Verification items for the finished model (mm, model axes). Round coordinates to 2 decimals unless told otherwise and drop trailing zeros. Loops run counter-clockwise (first coordinate to the right, second up) from the corner with the lowest first, then second, coordinate; pieces in that order, holes last. Notation, with made-up numbers: (-2, 68.5) - (33, 68.5) arc R27 ccw to (33, 90.5) - close; hole circle Ø3 at (79.5, -15.75). An arc over 180 degrees is marked (long way). Use a Markdown table: item, result. Add a question column.
```python
from build123d import *

# Parameters (mm, degrees)
SKETCH1_W          = 187.325
SKETCH1_H          = 332.057083461
EXTRUDE1_DEPTH     = 4.7625
CUT_EXTRUDE1_REACH = 264.098
CUT_EXTRUDE2_REACH = 264.098
SKETCH3_R          = 47.625
SKETCH3_R_2        = 8.5328125
FILLET1_R          = 6.35
CUT_EXTRUDE3_REACH = 264.098
SKETCH4_W          = 4.7625
SKETCH4_H          = 98.425


with BuildPart() as part:
    # Sketch1 → Extrude1 (new body)
    with BuildSketch(Plane.XY):
        with Locations((0, -78.716041731)):
            Rectangle(SKETCH1_W, SKETCH1_H)
    extrude(amount=-EXTRUDE1_DEPTH)

    # Sketch2 → Cut-Extrude1 (cut, up to next)
    with BuildSketch(Plane.XY, mode=Mode.PRIVATE) as cut_extrude1_sk1:
        with BuildLine():
            Line((-22.225, -203.2), (-22.225, -177.8))
            ThreePointArc((-22.225, -177.8), (0, -155.575), (22.225, -177.8))
            Line((22.225, -177.8), (22.225, -203.2))
            ThreePointArc((22.225, -203.2), (0, -225.425), (-22.225, -203.2))
        make_face()
    cut_extrude1_tool1 = extrude(cut_extrude1_sk1.sketch, amount=-CUT_EXTRUDE1_REACH, mode=Mode.PRIVATE) & part.part
    # Sketch2 → Cut-Extrude1 (cut, up to next)
    with BuildSketch(Plane.XY, mode=Mode.PRIVATE) as cut_extrude1_sk2:
        with BuildLine():
            Line((49.99355, -108.9152), (49.99355, -134.3152))
            ThreePointArc((49.99355, -134.3152), (46.0248, -138.28395), (42.05605, -134.3152))
            Line((42.05605, -134.3152), (42.05605, -108.9152))
            ThreePointArc((42.05605, -108.9152), (46.0248, -104.94645), (49.99355, -108.9152))
        make_face()
    cut_extrude1_tool2 = extrude(cut_extrude1_sk2.sketch, amount=-CUT_EXTRUDE1_REACH, mode=Mode.PRIVATE) & part.part
    # Sketch2 → Cut-Extrude1 (cut, up to next)
    with BuildSketch(Plane.XY, mode=Mode.PRIVATE) as cut_extrude1_sk3:
        with BuildLine():
            Line((-42.05605, -108.9152), (-42.05605, -134.3152))
            ThreePointArc((-42.05605, -134.3152), (-46.0248, -138.28395), (-49.99355, -134.3152))
            Line((-49.99355, -134.3152), (-49.99355, -108.9152))
            ThreePointArc((-49.99355, -108.9152), (-46.0248, -104.94645), (-42.05605, -108.9152))
        make_face()
    cut_extrude1_tool3 = extrude(cut_extrude1_sk3.sketch, amount=-CUT_EXTRUDE1_REACH, mode=Mode.PRIVATE) & part.part
    # Sketch2 → Cut-Extrude1 (cut, up to next)
    with BuildSketch(Plane.XY, mode=Mode.PRIVATE) as cut_extrude1_sk4:
        with BuildLine():
            Line((49.99355, -200.9648), (49.99355, -226.3648))
            ThreePointArc((49.99355, -226.3648), (46.0248, -230.33355), (42.05605, -226.3648))
            Line((42.05605, -226.3648), (42.05605, -200.9648))
            ThreePointArc((42.05605, -200.9648), (46.0248, -196.99605), (49.99355, -200.9648))
        make_face()
    cut_extrude1_tool4 = extrude(cut_extrude1_sk4.sketch, amount=-CUT_EXTRUDE1_REACH, mode=Mode.PRIVATE) & part.part
    # Sketch2 → Cut-Extrude1 (cut, up to next)
    with BuildSketch(Plane.XY, mode=Mode.PRIVATE) as cut_extrude1_sk5:
        with BuildLine():
            Line((-42.05605, -200.9648), (-42.05605, -226.3648))
            ThreePointArc((-42.05605, -226.3648), (-46.0248, -230.33355), (-49.99355, -226.3648))
            Line((-49.99355, -226.3648), (-49.99355, -200.9648))
            ThreePointArc((-49.99355, -200.9648), (-46.0248, -196.99605), (-42.05605, -200.9648))
        make_face()
    cut_extrude1_tool5 = extrude(cut_extrude1_sk5.sketch, amount=-CUT_EXTRUDE1_REACH, mode=Mode.PRIVATE) & part.part
    add(cut_extrude1_tool1.solids().sort_by_distance((0, -190.5, 0))[0], mode=Mode.SUBTRACT)
    add(cut_extrude1_tool2.solids().sort_by_distance((46.0248, -121.6152, 0))[0], mode=Mode.SUBTRACT)
    add(cut_extrude1_tool3.solids().sort_by_distance((-46.0248, -121.6152, 0))[0], mode=Mode.SUBTRACT)
    add(cut_extrude1_tool4.solids().sort_by_distance((46.0248, -213.6648, 0))[0], mode=Mode.SUBTRACT)
    add(cut_extrude1_tool5.solids().sort_by_distance((-46.0248, -213.6648, 0))[0], mode=Mode.SUBTRACT)

    # Sketch3 → Cut-Extrude2 (cut, up to next)
    with BuildSketch(Plane(origin=(0, 0, 0), x_dir=(-1, 0, 0), z_dir=(0, 0, -1)), mode=Mode.PRIVATE) as cut_extrude2_sk1:
        Circle(SKETCH3_R)
    cut_extrude2_tool1 = extrude(cut_extrude2_sk1.sketch, amount=CUT_EXTRUDE2_REACH, mode=Mode.PRIVATE) & part.part
    # Sketch3 → Cut-Extrude2 (cut, up to next)
    with BuildSketch(Plane(origin=(0, 0, 0), x_dir=(-1, 0, 0), z_dir=(0, 0, -1)), mode=Mode.PRIVATE) as cut_extrude2_sk2:
        with Locations((65.0875, 65.0875)):
            Circle(SKETCH3_R_2)
    cut_extrude2_tool2 = extrude(cut_extrude2_sk2.sketch, amount=CUT_EXTRUDE2_REACH, mode=Mode.PRIVATE) & part.part
    # Sketch3 → Cut-Extrude2 (cut, up to next)
    with BuildSketch(Plane(origin=(0, 0, 0), x_dir=(-1, 0, 0), z_dir=(0, 0, -1)), mode=Mode.PRIVATE) as cut_extrude2_sk3:
        with Locations((-65.0875, 65.0875)):
            Circle(SKETCH3_R_2)
    cut_extrude2_tool3 = extrude(cut_extrude2_sk3.sketch, amount=CUT_EXTRUDE2_REACH, mode=Mode.PRIVATE) & part.part
    # Sketch3 → Cut-Extrude2 (cut, up to next)
    with BuildSketch(Plane(origin=(0, 0, 0), x_dir=(-1, 0, 0), z_dir=(0, 0, -1)), mode=Mode.PRIVATE) as cut_extrude2_sk4:
        with Locations((-65.0875, -65.0875)):
            Circle(SKETCH3_R_2)
    cut_extrude2_tool4 = extrude(cut_extrude2_sk4.sketch, amount=CUT_EXTRUDE2_REACH, mode=Mode.PRIVATE) & part.part
    # Sketch3 → Cut-Extrude2 (cut, up to next)
    with BuildSketch(Plane(origin=(0, 0, 0), x_dir=(-1, 0, 0), z_dir=(0, 0, -1)), mode=Mode.PRIVATE) as cut_extrude2_sk5:
        with Locations((65.0875, -65.0875)):
            Circle(SKETCH3_R_2)
    cut_extrude2_tool5 = extrude(cut_extrude2_sk5.sketch, amount=CUT_EXTRUDE2_REACH, mode=Mode.PRIVATE) & part.part
    add(cut_extrude2_tool1.solids().sort_by_distance((0, 0, 0))[0], mode=Mode.SUBTRACT)
    add(cut_extrude2_tool2.solids().sort_by_distance((-65.0875, 65.0875, 0))[0], mode=Mode.SUBTRACT)
    add(cut_extrude2_tool3.solids().sort_by_distance((65.0875, 65.0875, 0))[0], mode=Mode.SUBTRACT)
    add(cut_extrude2_tool4.solids().sort_by_distance((65.0875, -65.0875, 0))[0], mode=Mode.SUBTRACT)
    add(cut_extrude2_tool5.solids().sort_by_distance((-65.0875, -65.0875, 0))[0], mode=Mode.SUBTRACT)

    # Fillet1
    fillet1_edges = [part.edges().sort_by_distance(p)[0] for p in [
        (93.6625, -244.744583461, -2.38125),
        (-93.6625, -244.744583461, -2.38125),
        (-93.6625, 87.3125, -2.38125),
        (93.6625, 87.3125, -2.38125),
    ]]
    fillet(fillet1_edges, radius=FILLET1_R)

    # Sketch4 → Cut-Extrude3 (cut, up to next)
    with BuildSketch(Plane(origin=(0, 0, -4.7625), x_dir=(-1, 0, 0), z_dir=(0, 0, -1)), mode=Mode.PRIVATE) as cut_extrude3_sk1:
        with Locations((-91.28125, 0)):
            Rectangle(SKETCH4_W, SKETCH4_H)
    cut_extrude3_tool1 = extrude(cut_extrude3_sk1.sketch, amount=-CUT_EXTRUDE3_REACH, mode=Mode.PRIVATE) & part.part
    # Sketch4 → Cut-Extrude3 (cut, up to next)
    with BuildSketch(Plane(origin=(0, 0, -4.7625), x_dir=(-1, 0, 0), z_dir=(0, 0, -1)), mode=Mode.PRIVATE) as cut_extrude3_sk2:
        with Locations((-91.28125, -157.432083461)):
            Rectangle(SKETCH4_W, SKETCH4_H)
    cut_extrude3_tool2 = extrude(cut_extrude3_sk2.sketch, amount=-CUT_EXTRUDE3_REACH, mode=Mode.PRIVATE) & part.part
    cut_extrude3_1 = cut_extrude3_tool1.solids().sort_by_distance((91.28125, 0, -4.7625))[0]
    add(cut_extrude3_1, mode=Mode.SUBTRACT)
    cut_extrude3_2 = cut_extrude3_tool2.solids().sort_by_distance((91.28125, -157.432083, -4.7625))[0]
    add(cut_extrude3_2, mode=Mode.SUBTRACT)
    cut_extrude3 = cut_extrude3_1 + cut_extrude3_2  # Cut-Extrude3 as one shape, for the pattern or mirror that repeats it

    # Mirror1: Cut-Extrude3 across plane
    add(cut_extrude3.mirror(Plane(origin=(0, 0, 0), x_dir=(0, 0, 1), z_dir=(1, 0, 0))), mode=Mode.SUBTRACT)


solid = part.part
```
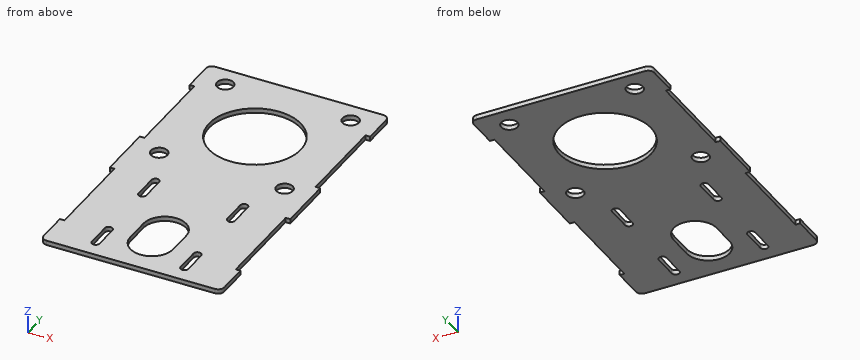
Q1. Section check D-D on x = 60. Record the cut outline in (y, z).
Q2. Thickness scan on line 1 along X through (y, z) = (-209, -3.5); line 2 along X through (y, z) = (-123, -3.5); line 3 along Y through (x, z) = (0, -2.5) (1 decimal). Record the ranges inside material, lowest first.
Q3. Section check B-B on y = 0. Record the cut outline in (x, z) (1 decimal).
Q4. Go/stop test with flat-tipped pins: pin 1 Ø1.4 at (y, z) = (-179, -3.5) entering from +X; pin 2 Ø13.5 at (x, y) = (65.09, 65.09) entering from -Z; pin 3 Ø1.4 at (x, z) = (90.5, -1.5) entering from +Y (3 decimals); pin 4 Ø1.4 at (y, z) = (8, -2.5) entering from -X. Record where each tip stops, or that it passes through.
Q5. Section check A-A on x = 0. Record the cut outline in (y, z) (1 decimal), plus the area to 3 significant figures.
Q6. Section check C-C on y = -152.5. Record the cut outline in (x, z), plus the area to 3 significant figures.
Determined:
| question | item | result |
|---|---|---|
| 1 | outline | (-244.74, -4.76) - (-71.94, -4.76) - (-71.94, 0) - (-244.74, 0) - close; (-58.24, -4.76) - (58.24, -4.76) - (58.24, 0) - (-58.24, 0) - close; (71.94, -4.76) - (87.31, -4.76) - (87.31, 0) - (71.94, 0) - close |
| 2 | line 1 | x = -93.66 to -49.99, -42.06 to -21.45, 21.45 to 42.06, 49.99 to 93.66 |
| 2 | line 2 | x = -88.9 to -49.99, -42.06 to 42.06, 49.99 to 88.9 |
| 2 | line 3 | y = -244.7 to -225.4, -155.6 to -47.6, 47.6 to 87.3 |
| 3 | outline | (-88.9, -4.8) - (-47.6, -4.8) - (-47.6, 0) - (-88.9, 0) - close; (47.6, -4.8) - (88.9, -4.8) - (88.9, 0) - (47.6, 0) - close |
| 4 | pin 1 | stops at x = 88.9 |
| 4 | pin 2 | passes through |
| 4 | pin 3 | stops at y = 86.805 |
| 4 | pin 4 | stops at x = -88.9 |
| 5 | outline | (-244.7, -4.8) - (-225.4, -4.8) - (-225.4, 0) - (-244.7, 0) - close; (-155.6, -4.8) - (-47.6, -4.8) - (-47.6, 0) - (-155.6, 0) - close; (47.6, -4.8) - (87.3, -4.8) - (87.3, 0) - (47.6, 0) - close |
| 5 | area | 795 mm² |
| 6 | outline | (-88.9, -4.76) - (88.9, -4.76) - (88.9, 0) - (-88.9, 0) - close |
| 6 | area | 847 mm² |
